```python
from build123d import *

# Parameters (mm, degrees)
BOSS_EXTRUDE1_DEPTH = 1
SKETCH4_W           = 40
SKETCH4_H           = 1
BOSS_EXTRUDE2_DEPTH = 30
SKETCH5_R           = 5
CUT_EXTRUDE1_DEPTH  = 47


with BuildPart() as part:
    # Sketch3 → Boss-Extrude1 (new body)
    with BuildSketch(Plane.XY):
        with BuildLine():
            Line((-20, 0), (-20, -15.25))
            Line((-20, -15.25), (20, -15.25))
            Line((20, -15.25), (20, 0))
            ThreePointArc((20, 0), (0, 20), (-20, 0))
        make_face()
    extrude(amount=BOSS_EXTRUDE1_DEPTH)

    # Sketch4 → Boss-Extrude2 (add)
    with BuildSketch(Plane.XY.offset(1)):
        with Locations((0, -15.75)):
            Rectangle(SKETCH4_W, SKETCH4_H)
    extrude(amount=-BOSS_EXTRUDE2_DEPTH)

    # Sketch5 → Cut-Extrude1 (cut)
    with BuildSketch(Plane.XY.offset(1)):
        with Locations((0, 1.5)):
            Circle(SKETCH5_R)
    extrude(amount=-CUT_EXTRUDE1_DEPTH, mode=Mode.SUBTRACT)


solid = part.part
```
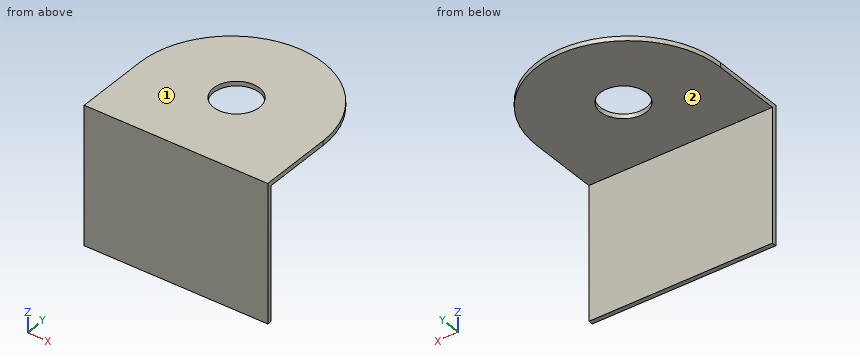
Check sheet for the modelled part. Datum: model origin and axes. Units: mm. Face numbers are marked on the shaded views. A direction names the side the tool comes from. Give positions to 0.01 mm unless a question says otherwise; leave off trailing zeros. Loops run counter-clockwise (first coordinate to the right, second up) from the corner with the lowest first, then second, coordinate; pieces in that order, holes last. Notation, with made-up numbers: M 43,2 L 64,2 A26 cw 64,37 Z; hole C 77,56 d4. An arc over 180 degrees is marked long. Answer in a Markdown table with one row per item.
1) Thickness scan on line 1 (Y direction, x = 0, z = 0.35); line 2 (Z direction, x = 2, y = 10); line 3 (Y direction, x = 7.5, z = -3.25). Record the ranges inside material, lowest first.
Solutions:
| item | result |
|---|---|
| line 1 | y = -16.25 to -3.5, 6.5 to 20 |
| line 2 | z = 0 to 1 |
| line 3 | y = -16.25 to -15.25 |
2) Cross-section at D-D (y = 1.5). Enter the section's corners in (x, z), plus the area to 3 significant figures.
Solutions:
| item | result |
|---|---|
| outline | M -19.94,0 L -5,0 L -5,1 L -19.94,1 Z; M 5,0 L 19.94,0 L 19.94,1 L 5,1 Z |
| area | 29.9 mm^2 |
3) Tool access check on the marked faces 1 and 2. Record the directions out of +Z, -Z, +X, -X, +Y, -Y that give a thin tool (end or side, any length) a straight path to the whole face; none if there is none.
Solutions:
| item | result |
|---|---|
| face 1 | +Z, +X, -X, +Y, -Y |
| face 2 | -Z, +X, -X, +Y |
4) Cross-section at A-A (y = -2.5). Enter the section's corners in (x, z).
Solutions:
| item | result |
|---|---|
| outline | M -20,0 L -3,0 L -3,1 L -20,1 Z; M 3,0 L 20,0 L 20,1 L 3,1 Z |
5) Cross-section at B-B (x = 0). Enter the section's corners in (y, z), plus the area to 4 significant figures.
Solutions:
| item | result |
|---|---|
| outline | M -16.25,-29 L -15.25,-29 L -15.25,0 L -3.5,0 L -3.5,1 L -16.25,1 Z; M 6.5,0 L 20,0 L 20,1 L 6.5,1 Z |
| area | 55.25 mm^2 |
6) Depth check by flat-ended pin: pin 1 (12 mm diameter, centred on y = 15.5, z = -10.5, fed in from -X); pin 2 (12 mm diameter, centred on x = 11, z = -8, fed in from +Y); pin 3 (4 mm diameter, centred on x = -11.5, y = -3, fed in from -Z). Enter the tip coordinate at first touch or a pass-through.
Solutions:
| item | result |
|---|---|
| pin 1 | passes through |
| pin 2 | stops at y = -15.25 |
| pin 3 | stops at z = 0 |
7) Cross-section at C-C (z = -5). Enter the section's corners in (x, y), plus the area to 3 significant figures.
Solutions:
| item | result |
|---|---|
| outline | M -20,-16.25 L 20,-16.25 L 20,-15.25 L -20,-15.25 Z |
| area | 40.0 mm^2 |
